Can you work these out from the model? Positions are in its coordinate system, mm. Face numbers are marked on the shaded views. A direction names the side the tool comes from. Round coordinates to 2 decimals unless told otherwise and drop trailing zeros. Write each loop counter-clockwise with the first axis right and the second up, starting at its lowest first coordinate (ties: lowest second). Pieces come first, ordered by that corner, then holes. Notation, with made-up numbers: M 59.5,38 L 66.5,38 A10 ccw 66.5,44 Z; hole C -11,42.5 d2. An arc over 180 degrees is marked long. Use one line per item in the form item = value. Start each with the question number.
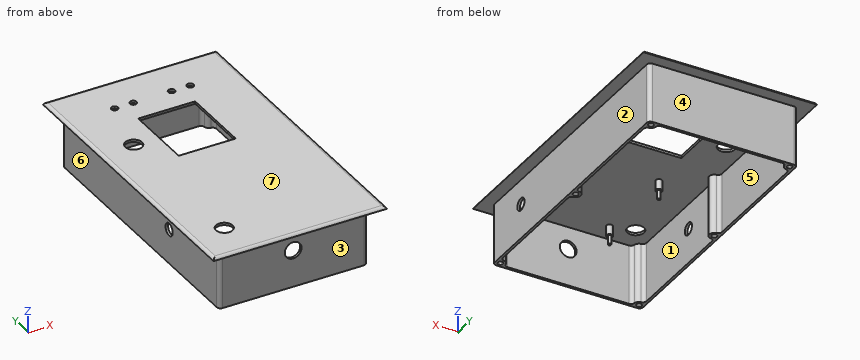
```python
from build123d import *

# Parameters (mm, degrees)
SKETCH1_W           = 120
SKETCH1_H           = 220
BOSS_EXTRUDE1_DEPTH = 48
SKETCH2_W           = 140
SKETCH2_H           = 240
BOSS_EXTRUDE2_DEPTH = 2
SHELL3_DEPTH        = 48
FILLET1_R           = 3
SKETCH4_R           = 2.75
SKETCH4_R_2         = 6.75
SKETCH4_W           = 46
SKETCH4_H           = 57
CUT_EXTRUDE1_DEPTH  = 147.982992213
SKETCH6_R           = 1.2
BOSS_EXTRUDE3_DEPTH = 15
SKETCH7_R           = 2.5
BOSS_EXTRUDE4_DEPTH = 8
CUT_EXTRUDE2_REACH  = 185.848
SKETCH9_R           = 5
CUT_EXTRUDE3_REACH  = 185.848
SKETCH10_R          = 5
CUT_EXTRUDE4_REACH  = 247.561
SKETCH11_R          = 6.75
FILLET2_R           = 3
FILLET3_R           = 3


# Read off the part's stored shape, not the designer's step: Ø3.0mm Dowel Hole1, Shell3
with BuildPart() as part:
    # Sketch1 → Boss-Extrude1 (new body)
    with BuildSketch(Plane.XY):
        Rectangle(SKETCH1_W, SKETCH1_H)
    extrude(amount=BOSS_EXTRUDE1_DEPTH)

    # Sketch2 → Boss-Extrude2 (add)
    with BuildSketch(Plane.XY.offset(48)):
        Rectangle(SKETCH2_W, SKETCH2_H)
    extrude(amount=BOSS_EXTRUDE2_DEPTH)

    # Ø3.0mm Dowel Hole1 outline → Ø3.0mm Dowel Hole1 (revolve, cut)
    with BuildSketch(Plane(origin=(-56, 0, 0), x_dir=(1, 0, 0), z_dir=(0, -1, 0))):
        Polygon((2.125, 48), (0, 49.276828815), (0, 0), (2.125, 0), align=None)
    revolve(axis=Axis((-56, 0, 0), (0, 0, 1)), mode=Mode.SUBTRACT)

    # 3.0mm Dowel Hole1 2 outline → 3.0mm Dowel Hole1 2 (revolve, cut)
    with BuildSketch(Plane(origin=(56, 0, 0), x_dir=(1, 0, 0), z_dir=(0, -1, 0))):
        Polygon((2.125, 48), (0, 49.276828815), (0, 0), (2.125, 0), align=None)
    revolve(axis=Axis((56, 0, 0), (0, 0, 1)), mode=Mode.SUBTRACT)

    # 3.0mm Dowel Hole1 3 outline → 3.0mm Dowel Hole1 3 (revolve, cut)
    with BuildSketch(Plane(origin=(-56, -106, 0), x_dir=(1, 0, 0), z_dir=(0, -1, 0))):
        Polygon((2.125, 48), (0, 49.276828815), (0, 0), (2.125, 0), align=None)
    revolve(axis=Axis((-56, -106, 0), (0, 0, 1)), mode=Mode.SUBTRACT)

    # 3.0mm Dowel Hole1 4 outline → 3.0mm Dowel Hole1 4 (revolve, cut)
    with BuildSketch(Plane(origin=(56, -106, 0), x_dir=(1, 0, 0), z_dir=(0, -1, 0))):
        Polygon((2.125, 48), (0, 49.276828815), (0, 0), (2.125, 0), align=None)
    revolve(axis=Axis((56, -106, 0), (0, 0, 1)), mode=Mode.SUBTRACT)

    # 3.0mm Dowel Hole1 5 outline → 3.0mm Dowel Hole1 5 (revolve, cut)
    with BuildSketch(Plane(origin=(-56, 106, 0), x_dir=(1, 0, 0), z_dir=(0, -1, 0))):
        Polygon((2.125, 48), (0, 49.276828815), (0, 0), (2.125, 0), align=None)
    revolve(axis=Axis((-56, 106, 0), (0, 0, 1)), mode=Mode.SUBTRACT)

    # 3.0mm Dowel Hole1 6 outline → 3.0mm Dowel Hole1 6 (revolve, cut)
    with BuildSketch(Plane(origin=(56, 106, 0), x_dir=(1, 0, 0), z_dir=(0, -1, 0))):
        Polygon((2.125, 48), (0, 49.276828815), (0, 0), (2.125, 0), align=None)
    revolve(axis=Axis((56, 106, 0), (0, 0, 1)), mode=Mode.SUBTRACT)

    # Shell3 outline → Shell3 (cut)
    with BuildSketch(Plane.XY):
        with BuildLine():
            Line((52.392282578, 108), (-52.392282578, 108))
            ThreePointArc((-52.392282578, 108), (-53.083184528, 103.083184528), (-58, 102.392282578))
            Line((-58, 102.392282578), (-58, 3.607717422))
            ThreePointArc((-58, 3.607717422), (-51.875, 0), (-58, -3.607717422))
            Line((-58, -3.607717422), (-58, -102.392282578))
            ThreePointArc((-58, -102.392282578), (-53.083184528, -103.083184528), (-52.392282578, -108))
            Line((-52.392282578, -108), (52.392282578, -108))
            ThreePointArc((52.392282578, -108), (53.083184528, -103.083184528), (58, -102.392282578))
            Line((58, -102.392282578), (58, -3.607717422))
            ThreePointArc((58, -3.607717422), (51.875, 0), (58, 3.607717422))
            Line((58, 3.607717422), (58, 102.392282578))
            ThreePointArc((58, 102.392282578), (53.083184528, 103.083184528), (52.392282578, 108))
        make_face()
    extrude(amount=SHELL3_DEPTH, mode=Mode.SUBTRACT)

    # Fillet1
    fillet1_edges = [part.edges().sort_by_distance(p)[0] for p in [
        (-52.392282578, 108, 24),
        (-58, 3.607717422, 24),
        (58, -3.607717422, 24),
        (52.392282578, -108, 24),
        (58, 102.392282578, 24),
        (-58, -102.392282578, 24),
        (-58, -3.607717422, 24),
        (58, 3.607717422, 24),
        (-52.392282578, -108, 24),
        (58, -102.392282578, 24),
        (-58, 102.392282578, 24),
        (52.392282578, 108, 24),
    ]]
    fillet(fillet1_edges, radius=FILLET1_R)

    # Sketch4 → Cut-Extrude1 (cut, through all)
    with BuildSketch(Plane(origin=(0, 0, 48), x_dir=(-1, 0, 0), z_dir=(0, 0, -1))):
        with Locations((15.5, 88)):
            Circle(SKETCH4_R)
        with Locations(Location((30.5, 88, 0), (0, 0, 180))):
            Circle(SKETCH4_R)
        with Locations((-30.5, 88)):
            Circle(SKETCH4_R)
        with Locations(Location((-15.5, 88, 0), (0, 0, 180))):
            Circle(SKETCH4_R)
        with Locations((43, 39.5)):
            Circle(SKETCH4_R_2)
        with Locations((43, -88)):
            Circle(SKETCH4_R_2)
        with Locations((0, 39.5)):
            Rectangle(SKETCH4_W, SKETCH4_H)
    extrude(amount=-CUT_EXTRUDE1_DEPTH, mode=Mode.SUBTRACT)

    # Sketch6 → Boss-Extrude3 (add)
    with BuildSketch(Plane(origin=(0, 0, 48), x_dir=(-1, 0, 0), z_dir=(0, 0, -1))):
        with Locations(Location((-45.079, -23.120003999, 0), (0, 0, 180))):
            Circle(SKETCH6_R)
        with Locations(Location((24.517, -23.120003999, 0), (0, 0, 180))):
            Circle(SKETCH6_R)
        with Locations(Location((-45.079, -92.589003999, 0), (0, 0, 180))):
            Circle(SKETCH6_R)
        with Locations(Location((24.517, -92.589003999, 0), (0, 0, 180))):
            Circle(SKETCH6_R)
    extrude(amount=BOSS_EXTRUDE3_DEPTH)

    # Sketch7 → Boss-Extrude4 (add)
    with BuildSketch(Plane(origin=(0, 0, 48), x_dir=(-1, 0, 0), z_dir=(0, 0, -1))):
        with Locations(Location((-45.079, -23.120003999, 0), (0, 0, 180))):
            Circle(SKETCH7_R)
        with Locations(Location((24.517, -23.120003999, 0), (0, 0, 180))):
            Circle(SKETCH7_R)
        with Locations(Location((24.517, -92.589003999, 0), (0, 0, 180))):
            Circle(SKETCH7_R)
        with Locations(Location((-45.079, -92.589003999, 0), (0, 0, 180))):
            Circle(SKETCH7_R)
    extrude(amount=BOSS_EXTRUDE4_DEPTH)

    # Sketch9 → Cut-Extrude2 (cut, up to next)
    with BuildSketch(Plane(origin=(60, 0, 0), x_dir=(0, 0, -1), z_dir=(1, 0, 0)), mode=Mode.PRIVATE) as cut_extrude2_sk1:
        with Locations((-28, -70)):
            Circle(SKETCH9_R)
    cut_extrude2_tool1 = extrude(cut_extrude2_sk1.sketch, amount=-CUT_EXTRUDE2_REACH, mode=Mode.PRIVATE) & part.part
    add(cut_extrude2_tool1.solids().sort_by_distance((60, -70, 28))[0], mode=Mode.SUBTRACT)

    # Sketch10 → Cut-Extrude3 (cut, up to next)
    with BuildSketch(Plane.ZY.offset(60), mode=Mode.PRIVATE) as cut_extrude3_sk1:
        with Locations((28, -40)):
            Circle(SKETCH10_R)
    cut_extrude3_tool1 = extrude(cut_extrude3_sk1.sketch, amount=-CUT_EXTRUDE3_REACH, mode=Mode.PRIVATE) & part.part
    add(cut_extrude3_tool1.solids().sort_by_distance((-60, -40, 28))[0], mode=Mode.SUBTRACT)

    # Sketch11 → Cut-Extrude4 (cut, up to next)
    with BuildSketch(Plane.XZ.offset(110), mode=Mode.PRIVATE) as cut_extrude4_sk1:
        with Locations(Location((0, 30, 0), (0, 0, 270))):
            Circle(SKETCH11_R)
    cut_extrude4_tool1 = extrude(cut_extrude4_sk1.sketch, amount=-CUT_EXTRUDE4_REACH, mode=Mode.PRIVATE) & part.part
    add(cut_extrude4_tool1.solids().sort_by_distance((0, -110, 30))[0], mode=Mode.SUBTRACT)

    # Fillet2
    fillet2_edges = [part.edges().sort_by_distance(p)[0] for p in [
        (60, -110, 24),
        (-60, -110, 24),
        (-60, 110, 24),
        (60, 110, 24),
    ]]
    fillet(fillet2_edges, radius=FILLET2_R)

    # Fillet3
    # the kernel refuses this fillet: 3 mm, written as the material it takes off along each edge
    with BuildSketch(Plane(origin=(77.071067812, -120, 50), x_dir=(0, 0, -1), z_dir=(-1, 0, 0)), Plane(origin=(-77.071067812, 120, 50), x_dir=(0, 0, -1), z_dir=(1, 0, 0))) as fillet3_piece_1:
        with BuildLine():
            CenterArc((3, -2.828427125), FILLET3_R, 109.471220634, 70.528779366)
            Line((0, -2.828427125), (-0.06, -2.828427125))
            Line((-0.06, -2.828427125), (-0.06, 0))
            Line((-0.06, 0), (0, 0.06))
            ThreePointArc((0, 0.06), (1, 0.06), (1.98, 0.056568542))
            Line((1.98, 0.056568542), (2, 0))
        make_face()
    extrude(amount=154.142135624, mode=Mode.SUBTRACT)
    with BuildSketch(Plane(origin=(-70, -127.071067812, 50), x_dir=(0, 0, -1), z_dir=(0, 1, 0)), Plane(origin=(70, 127.071067812, 50), x_dir=(0, 0, -1), z_dir=(0, -1, 0))) as fillet3_piece_2:
        with BuildLine():
            CenterArc((3, -2.828427125), FILLET3_R, 109.471220634, 70.528779366)
            Line((0, -2.828427125), (-0.06, -2.828427125))
            Line((-0.06, -2.828427125), (-0.06, 0))
            Line((-0.06, 0), (0, 0.06))
            ThreePointArc((0, 0.06), (1, 0.06), (1.98, 0.056568542))
            Line((1.98, 0.056568542), (2, 0))
        make_face()
    extrude(amount=254.142135624, mode=Mode.SUBTRACT)


solid = part.part
```
1. Which directions (+Z, -Z, +X, -X, +Y, -Y) give clear straight access to the entire face, cutting with the end or side of a thin tool? Please do the marked faces 4, 5, 6 and 7.
2. If we section it at B-B (x = -15.5): List the corners of the cut face in (y, z) for me.
3. If we section it at A-A (y = 88): List the corners of the cut face in (x, z) for me.
4. If we section it at D-D (y = 25): List the corners of the cut face in (x, z) for me, and give its area (3 significant figures).
5. Please list where these lines run through material, in increasing order: line 1 along X through (y, z) = (-80.5, 6); line 2 along Y through (x, z) = (4, 39); line 3 along Y through (x, z) = (56, 35) (3 decimals).
6. Will these pins go through, and if not, where does the flat tip stop? pin 1 (24 mm diameter, centred on x = -19.5, z = 13, fed in from +Y); pin 2 (14.5 mm diameter, centred on y = 45, z = 15.5, fed in from -X); pin 3 (2.5 mm diameter, centred on x = 44, y = -24, fed in from -Z).
7. If we mould it in two halves opening along Y, with no side actions, what happens to the marked faces 1, 2 and 3? For each: pulls with the +Y half, pulls with the -Y half, needs draft (parallel to the pull), parting line crosses it, or undercut.
8. If we section it at C-C (x = -30.5): List the corners of the cut face in (y, z) for me.
Model answer:
q1.face_4 = -Z, +X, -X, +Y
q1.face_5 = -Z
q1.face_6 = -Z, -X, +Y, -Y
q1.face_7 = +Z, +X, -X, +Y, -Y
q2.outline = M -120,48 L -110,48 L -110,0 L -108,0 L -108,48 L 11,48 L 11,50 L -117.17,50 A3 ccw Z; M 68,48 L 85.25,48 L 85.25,50 L 68,50 Z; M 90.75,48 L 108,48 L 108,0 L 110,0 L 110,48 L 120,48 A3 ccw 117.17,50 L 90.75,50 Z
q3.outline = M -70,48 L -60,48 L -60,0 L -58,0 L -58,48 L -33.25,48 L -33.25,50 L -67.17,50 A3 ccw Z; M -27.75,48 L -18.25,48 L -18.25,50 L -27.75,50 Z; M -12.75,48 L 12.75,48 L 12.75,50 L -12.75,50 Z; M 18.25,48 L 27.75,48 L 27.75,50 L 18.25,50 Z; M 33.25,48 L 58,48 L 58,0 L 60,0 L 60,48 L 70,48 A3 ccw 67.17,50 L 33.25,50 Z
q4.outline = M -70,48 L -60,48 L -60,0 L -58,0 L -58,48 L -23,48 L -23,50 L -67.17,50 A3 ccw Z; M 23,48 L 58,48 L 58,0 L 60,0 L 60,48 L 70,48 A3 ccw 67.17,50 L 23,50 Z
q4.area = 377 mm2
q5.line_1 = -60 to -58, 58 to 60
q5.line_2 = -110 to -108, 108 to 110
q5.line_3 = -110 to -108.125, -103.875 to -101.774, -4.226 to -2.125, 2.125 to 4.226, 101.774 to 103.875, 108.125 to 110
q6.pin_1 = 110
q6.pin_2 = -60
q6.pin_3 = 33
q7.face_1 = undercut
q7.face_2 = needs draft
q7.face_3 = pulls with the -Y half
q8.outline = M -120,48 L -110,48 L -110,0 L -108,0 L -108,48 L 85.25,48 L 85.25,50 L -117.17,50 A3 ccw Z; M 90.75,48 L 108,48 L 108,0 L 110,0 L 110,48 L 120,48 A3 ccw 117.17,50 L 90.75,50 Z
